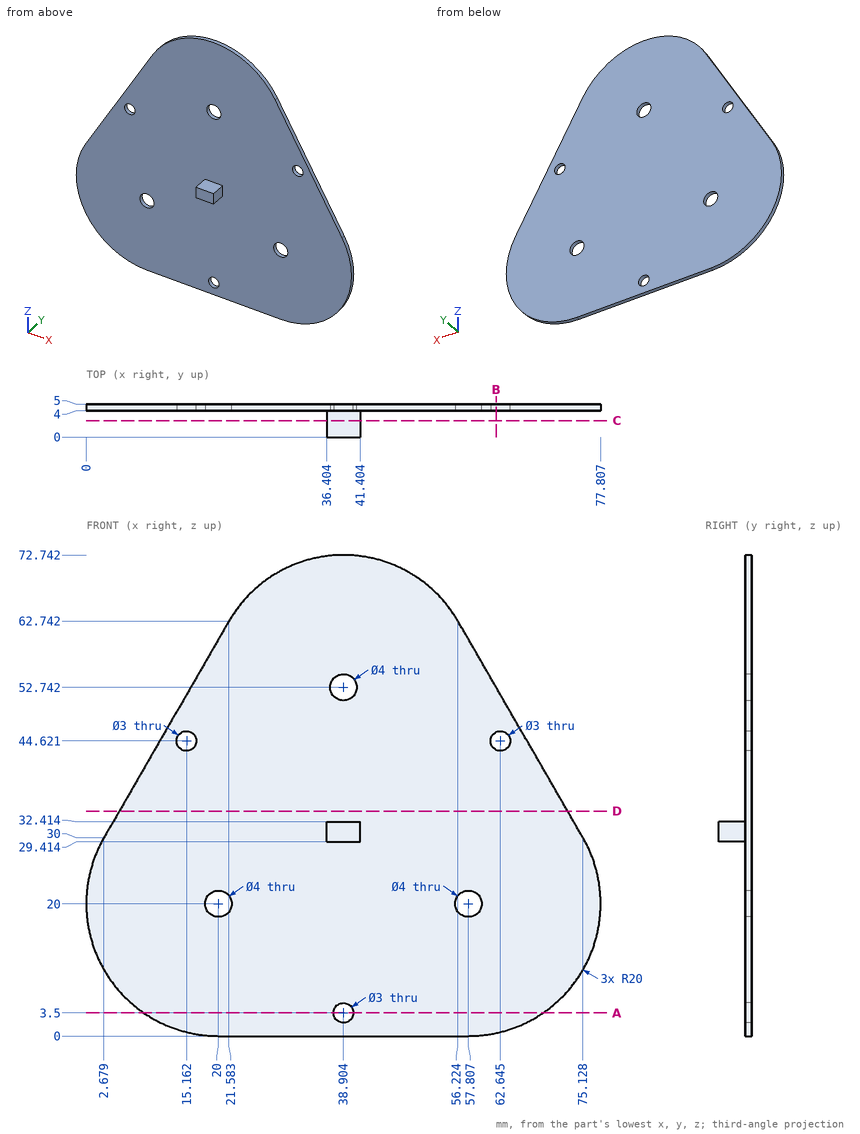
Job drawing, mm, ordinate dimensions from the low corner. One solid piece. Round coordinates to 2 decimals unless told otherwise and drop trailing zeros. Write each loop counter-clockwise with the first axis right and the second up, starting at its lowest first coordinate (ties: lowest second). Pieces come first, ordered by that corner, then holes.
1) Band-saw the part on D-D, the plane z = 34. List the corners of the cut face in (x, y).
2) Band-saw the part on A-A, the plane z = 3.5. List the corners of the cut face in (x, y).
3) Band-saw the part on B-B, the plane x = 62. List the corners of the cut face in (y, z) (1 decimal).
4) Drill centre lines: probe 1 along Y at (x, z) = (38, 9.5); probe 2 along X at (y, z) = (2.15, 30.5); probe 3 along Z at (x, y) = (19.5, 4.8) (1 decimal). Where is each one in solid material? Low to high.
5) Pin check, flat tips, straight feed: pin 1 (6.5 mm diameter, centred on x = 38.9, z = 52.74, fed in from -Y); pin 2 (2.5 mm diameter, centred on x = 38.9, z = 3.5, fed in from -Y); pin 3 (1.5 mm diameter, centred on y = 2, z = 30.5, fed in from +X); pin 4 (1.5 mm diameter, centred on x = 41.5, y = 1, fed in from -Z). Stop position of each tip, or through.
6) Band-saw the part on C-C, the plane y = 2.5. List the corners of the cut face in (x, z).
Ans:
1. outline: (4.99, 4) - (72.82, 4) - (72.82, 5) - (4.99, 5) - close
2. outline: (8.7, 4) - (37.4, 4) - (37.4, 5) - (8.7, 5) - close; (40.4, 4) - (69.11, 4) - (69.11, 5) - (40.4, 5) - close
3. outline: (4, 0.4) - (5, 0.4) - (5, 43.3) - (4, 43.3) - close; (4, 46) - (5, 46) - (5, 52.7) - (4, 52.7) - close
4. probe 1: y = 4 to 5
4. probe 2: x = 36.4 to 41.4
4. probe 3: z = 0 to 18.1, 21.9 to 59.1
5. pin 1: stops at y = 4
5. pin 2: passes through
5. pin 3: stops at x = 41.4
5. pin 4: stops at z = 29.41
6. outline: (36.4, 29.41) - (41.4, 29.41) - (41.4, 32.41) - (36.4, 32.41) - close
